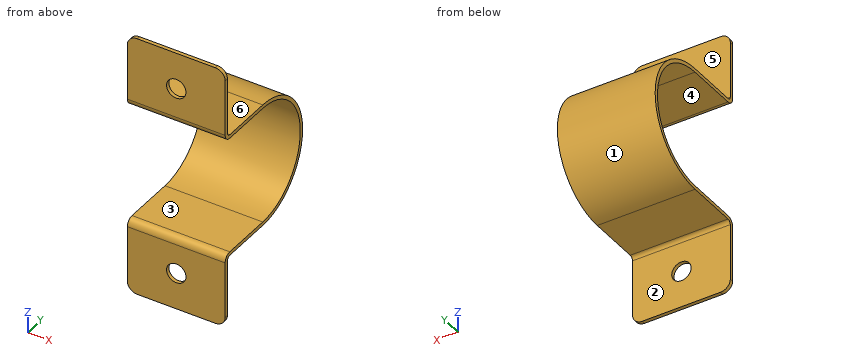
from build123d import *

# Parameters (mm, degrees)
BASE_FLANGE1_DEPTH = 10
SKETCH6_R          = 1.984375
CUT_EXTRUDE1_DEPTH = 38.483329628
FILLET1_R          = 2
FILLET2_R          = 2
FILLET3_R          = 2


# Sheet-metal steps are written as plain solids
with BuildPart() as part:
    # Sketch1 → Base-Flange1 (new, symmetric)
    with BuildSketch(Plane(origin=(0, 0, 0), x_dir=(0, 0, -1), z_dir=(1, 0, 0))):
        with BuildLine():
            Line((-27, 0), (-13.4732, 0))
            ThreePointArc((-13.4732, 0), (-12.43149029, 0.43149029), (-12, 1.4732))
            Line((-12, 1.4732), (-12, 12))
            ThreePointArc((-12, 12), (0, 24), (12, 12))
            Line((12, 12), (12, 1.4732))
            ThreePointArc((12, 1.4732), (12.43149029, 0.43149029), (13.4732, 0))
            Line((13.4732, 0), (27, 0))
            Line((27, 0), (27, 0.7366))
            Line((27, 0.7366), (13.4732, 0.7366))
            ThreePointArc((13.4732, 0.7366), (12.952345145, 0.952345145), (12.7366, 1.4732))
            Line((12.7366, 1.4732), (12.7366, 12))
            ThreePointArc((12.7366, 12), (0, 24.7366), (-12.7366, 12))
            Line((-12.7366, 12), (-12.7366, 1.4732))
            ThreePointArc((-12.7366, 1.4732), (-12.952345145, 0.952345145), (-13.4732, 0.7366))
            Line((-13.4732, 0.7366), (-27, 0.7366))
            Line((-27, 0.7366), (-27, 0))
        make_face()
    extrude(amount=BASE_FLANGE1_DEPTH, both=True)

    # Sketch6 → Cut-Extrude1 (cut, through all)
    with BuildSketch(Plane(origin=(0, 0.7366, 0), x_dir=(1, 0, 0), z_dir=(0, 1, 0))):
        with Locations(Location((0, -19.5, 0), (0, 0, 270))):
            Circle(SKETCH6_R)
    cut_extrude1 = extrude(amount=-CUT_EXTRUDE1_DEPTH, mode=Mode.SUBTRACT)

    # Mirror1: Cut-Extrude1 across plane
    add(cut_extrude1.mirror(Plane.XY), mode=Mode.SUBTRACT)

    # Fillet1
    fillet1_edges = [part.edges().sort_by_distance(p)[0] for p in [
        (10, 0.3683, -27),
    ]]
    fillet(fillet1_edges, radius=FILLET1_R)

    # Fillet2
    fillet2_edges = [part.edges().sort_by_distance(p)[0] for p in [
        (-10, 0.3683, -27),
    ]]
    fillet(fillet2_edges, radius=FILLET2_R)

    # Fillet3
    fillet3_edges = [part.edges().sort_by_distance(p)[0] for p in [
        (-10, 0.3683, 27),
        (10, 0.3683, 27),
    ]]
    fillet(fillet3_edges, radius=FILLET3_R)


solid = part.part
Geometry check sheet. Reference: the model listing, model coordinates, mm. Face numbers are marked on the shaded views. A direction names the side the tool comes from. Give positions to 0.01 mm unless a question says otherwise; leave off trailing zeros. Write each loop counter-clockwise with the first axis right and the second up, starting at its lowest first coordinate (ties: lowest second). Pieces come first, ordered by that corner, then holes.
1) Thickness scan on line 1 (X direction, y = 0.6, z = -19.5); line 2 (Z direction, x = -6.25, y = 11.75); line 3 (Y direction, x = 1, z = 16.5). Record the ranges inside material, lowest first.
Values follow:
line 1: x = -10 to -1.98, 1.98 to 10
line 2: z = -12.74 to -12, 12 to 12.74
line 3: y = 0 to 0.74
2) Set-up check for the marked faces 1, 2 and 3: record each of +Z, -Z, +X, -X, +Y, -Y from which the full face is reachable in a straight line by a thin tool's end or side.
Values follow:
face 1: +X, -X, +Y
face 2: -Z, +X, -X, +Y
face 3: +X, -X, -Y
3) Release check for a two-part mould opening along Z. For the marked faces 4, 5 and 6 record: released by +Z, released by -Z, zero draft, split by the parting line, or undercut.
Values follow:
face 4: undercut
face 5: zero draft
face 6: released by +Z
4) Go/stop test with flat-tipped pins: pin 1 Ø5.5 at (x, y) = (1, 5.5) entering from +Z; pin 2 Ø3 at (y, z) = (7, 15.5) entering from -X; pin 3 Ø6 at (x, y) = (-1.5, 7.5) entering from -Z; pin 4 Ø3 at (x, z) = (7.5, 17.5) entering from +Y. Record where each tip stops, or that it passes through.
Values follow:
pin 1: stops at z = 12.74
pin 2: passes through
pin 3: stops at z = -12.74
pin 4: stops at y = 0.74
5) Cross-section at C-C (y = 13.75). Record the boundary of the cut face in (x, z).
Values follow:
outline: (-10, -12.62) - (10, -12.62) - (10, -11.87) - (-10, -11.87) - close; (-10, 11.87) - (10, 11.87) - (10, 12.62) - (-10, 12.62) - close
6) Cross-section at B-B (z = -19.5). Record the boundary of the cut face in (x, y), plus the area to 3 significant figures.
Values follow:
outline: (-10, 0) - (-1.98, 0) - (-1.98, 0.74) - (-10, 0.74) - close; (1.98, 0) - (10, 0) - (10, 0.74) - (1.98, 0.74) - close
area: 11.8 mm2
7) Cross-section at A-A (x = 0). Record the boundary of the cut face in (y, z).
Values follow:
outline: (0, -27) - (0.74, -27) - (0.74, -21.48) - (0, -21.48) - close; (0, -17.52) - (0.74, -17.52) - (0.74, -13.47) arc R0.74 cw to (1.47, -12.74) - (12, -12.74) arc R12.74 ccw to (12, 12.74) - (1.47, 12.74) arc R0.74 cw to (0.74, 13.47) - (0.74, 17.52) - (0, 17.52) - (0, 13.47) arc R1.47 ccw to (1.47, 12) - (12, 12) arc R12 cw to (12, -12) - (1.47, -12) arc R1.47 ccw to (0, -13.47) - close; (0, 21.48) - (0.74, 21.48) - (0.74, 27) - (0, 27) - close
8) Cross-section at D-D (x = 4). Record the boundary of the cut face in (y, z).
Values follow:
outline: (0, -27) - (0.74, -27) - (0.74, -13.47) arc R0.74 cw to (1.47, -12.74) - (12, -12.74) arc R12.74 ccw to (12, 12.74) - (1.47, 12.74) arc R0.74 cw to (0.74, 13.47) - (0.74, 27) - (0, 27) - (0, 13.47) arc R1.47 ccw to (1.47, 12) - (12, 12) arc R12 cw to (12, -12) - (1.47, -12) arc R1.47 ccw to (0, -13.47) - close
